from build123d import *

# Parameters (mm, degrees)
SKETCH1_R                 = 50.8
BOSS_EXTRUDE1_DEPTH       = 3.175
SKETCH2_R                 = 38.1
BOSS_EXTRUDE2_DEPTH       = 9.525
F_2_CLEARANCE_HOLE1_D     = 2.4384
F_2_CLEARANCE_HOLE1_DEPTH = 25.4
F_2_CLEARANCE_HOLE1_TIP   = 0.732569267


with BuildPart() as part:
    # Sketch1 → Boss-Extrude1 (new body)
    with BuildSketch(Plane(origin=(0, 0, 0), x_dir=(1, 0, 0), z_dir=(0, 1, 0))):
        Circle(SKETCH1_R)
    extrude(amount=BOSS_EXTRUDE1_DEPTH)

    # Sketch2 → Boss-Extrude2 (add)
    with BuildSketch(Plane.XZ):
        Circle(SKETCH2_R)
    extrude(amount=BOSS_EXTRUDE2_DEPTH)

    # #2 Clearance Hole1
    with Locations(Plane(origin=(0, 3.175, 0), x_dir=(-1, 0, 0), z_dir=(0, 1, 0))):
        with Locations((0, -40.48125), (-40.48125, 0), (40.48125, 0), (0, 40.48125)):
            Hole(F_2_CLEARANCE_HOLE1_D / 2, depth=F_2_CLEARANCE_HOLE1_DEPTH)
            with Locations((0, 0, -(F_2_CLEARANCE_HOLE1_DEPTH + F_2_CLEARANCE_HOLE1_TIP / 2))):  # 118° drill point
                Cone(0, F_2_CLEARANCE_HOLE1_D / 2, F_2_CLEARANCE_HOLE1_TIP, mode=Mode.SUBTRACT)


solid = part.part
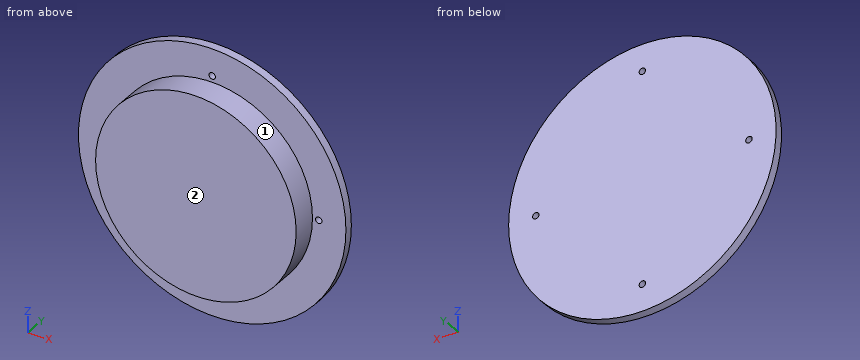
Here's how the part is built. I have some questions about the finished solid (model axes, mm). Face numbers are marked on the shaded views. A direction names the side the tool comes from. Coordinates: 2 decimals unless noted, no trailing zeros. Write each loop counter-clockwise with the first axis right and the second up, starting at its lowest first coordinate (ties: lowest second). Pieces come first, ordered by that corner, then holes.
Item 1: Will these pins go through, and if not, where does the flat tip stop? pin 1 (2 mm diameter, centred on x = -40.48, z = 0, fed in from -Y); pin 2 (5 mm diameter, centred on y = 1.5, z = 31.5, fed in from -X); pin 3 (1.5 mm diameter, centred on x = -29.5, y = -6, fed in from +Z); pin 4 (4 mm diameter, centred on x = 40.48, z = 0, fed in from -Y).
Item 2: On a 3-axis mill with a long thin cutter (end or side, diameter ignored), from which of +Z, -Z, +X, -X, +Y, -Y can I reach the whole of each face in a straight line? I mean the marked faces 1 and 2. Say none if no direction works.
Item 3: If I drill on line 1 (Z direction, x = 0, y = 1.8); line 2 (Y direction, x = -43.5, z = -17) (3 decimals); line 3 (X direction, y = -1.5, z = -4), over which ranges is the centre line in solid material (lowest first)?
Item 4: I want a section at A-A on z = 0. Write out the boundary of the cut face in (x, y) (3 decimals), and give its area (3 significant figures).
Item 5: I want a section at B-B on x = 0. Write out the boundary of the cut face in (y, z) (3 decimals), and give its area (3 significant figures).
Item 6: I want a section at C-C on x = -35.5. Write out the boundary of the cut face in (y, z) (3 decimals).
Item 7: I want a section at D-D on z = -14. Write out the boundary of the cut face in (x, y) (3 decimals), and give its area (3 significant figures).
Findings below:
1. pin 1: passes through
1. pin 2: stops at x = -41.71
1. pin 3: stops at z = 25
1. pin 4: stops at y = 0
2. face 1: -Y
2. face 2: +Z, -Z, +X, -X, -Y
3. line 1: z = -50.8 to -41.7, -39.26 to 39.26, 41.7 to 50.8
3. line 2: y = 0 to 3.175
3. line 3: x = -37.89 to 37.89
4. outline: (-50.8, 0) - (-41.7, 0) - (-41.7, 3.175) - (-50.8, 3.175) - close; (-39.262, 0) - (-38.1, 0) - (-38.1, -9.525) - (38.1, -9.525) - (38.1, 0) - (39.262, 0) - (39.262, 3.175) - (-39.262, 3.175) - close; (41.7, 0) - (50.8, 0) - (50.8, 3.175) - (41.7, 3.175) - close
4. area: 1,030 mm2
5. outline: (-9.525, -38.1) - (0, -38.1) - (0, -39.262) - (3.175, -39.262) - (3.175, 39.262) - (0, 39.262) - (0, 38.1) - (-9.525, 38.1) - close; (0, -50.8) - (3.175, -50.8) - (3.175, -41.7) - (0, -41.7) - close; (0, 41.7) - (3.175, 41.7) - (3.175, 50.8) - (0, 50.8) - close
5. area: 1,030 mm2
6. outline: (-9.525, -13.833) - (0, -13.833) - (0, -36.337) - (3.175, -36.337) - (3.175, 36.337) - (0, 36.337) - (0, 13.833) - (-9.525, 13.833) - close
7. outline: (-48.833, 0) - (-35.435, 0) - (-35.435, -9.525) - (35.435, -9.525) - (35.435, 0) - (48.833, 0) - (48.833, 3.175) - (-48.833, 3.175) - close
7. area: 985 mm2
